Model file for the job. Use its own axes, mm. Coordinates: 2 decimals unless noted, no trailing zeros. Order: outer loops, then holes, each group sorted by start corner. A loop starts at its lowest first (then second) coordinate and runs counter-clockwise, first axis right, second up. Notation, with made-up numbers: (-19.5, -11.75) -> (8.5, -11.75) arc R35 ccw to (8.5, 25.25) -> close; hole circle Ø5 at (86, 32). An arc over 180 degrees is marked (long way). Write item = value, one per line. Start each with the question number.
Q1. Cut at D-D, the plane y = 1.45. Give the number of separate pieces and of enclosed holes in the cut face, plus the area to 3 significant figures.
Q2. Cut at A-A, the plane x = -11.5. List the corners of the cut face in (y, z).
Q3. Flat gauge pin, fed straight in: pin 1 (1.8 mm diameter, centred on x = -29.13, z = -12, fed in from -Y). Where does the tip first touch, or does it go through?
Q4. Cut at C-C, the plane z = 5.25. List the corners of the cut face in (x, y).
Q5. Wall check: line 1 (Z direction, x = 13, y = 0.85); line 2 (X direction, y = 1.7, z = 7); line 3 (X direction, y = 0.65, z = 9.25). Give the ranges that are in metal, low to high. Write a range as from..to.
Q6. Cut at B-B, the plane z = 12. List the corners of the cut face in (x, y).
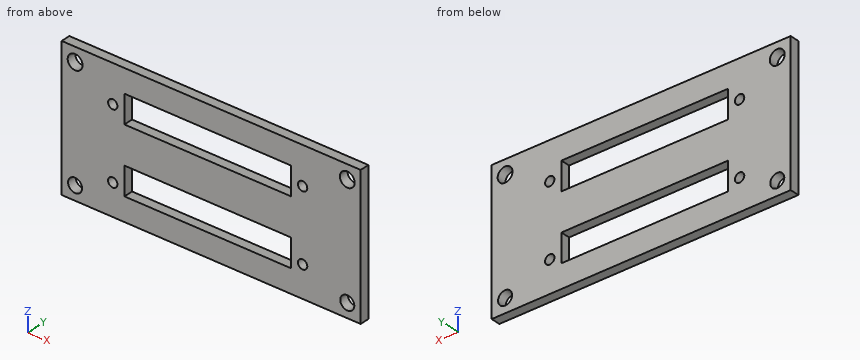
from build123d import *

# Parameters (mm, degrees)
SKETCH2_W           = 64
SKETCH2_H           = 30
SKETCH2_R           = 1.589304783
SKETCH2_R_2         = 1.5
BOSS_EXTRUDE1_DEPTH = 2
SKETCH3_R           = 1
SKETCH3_W           = 35.640445049
SKETCH3_H           = 6
CUT_EXTRUDE1_DEPTH  = 2


with BuildPart() as part:
    # Sketch2 → Boss-Extrude1 (new body)
    with BuildSketch(Plane(origin=(0, 0, 0), x_dir=(1, 0, 0), z_dir=(0, 1, 0))):
        Rectangle(SKETCH2_W, SKETCH2_H)
        with Locations(Location((-29.13, -12, 0), (0, 0, 270))):
            Circle(SKETCH2_R, mode=Mode.SUBTRACT)
        with Locations(Location((-29.134119409, 12, 0), (0, 0, 270))):
            Circle(SKETCH2_R_2, mode=Mode.SUBTRACT)
        with Locations(Location((29.13, -12, 0), (0, 0, 90))):
            Circle(SKETCH2_R, mode=Mode.SUBTRACT)
        with Locations(Location((29.134119409, 12, 0), (0, 0, 90))):
            Circle(SKETCH2_R_2, mode=Mode.SUBTRACT)
    extrude(amount=BOSS_EXTRUDE1_DEPTH)

    # Sketch3 → Cut-Extrude1 (cut)
    with BuildSketch(Plane(origin=(0, 2, 0), x_dir=(1, 0, 0), z_dir=(0, 1, 0))):
        with Locations(Location((-21.068550994, 8.267170413, 0), (0, 0, 270))):
            Circle(SKETCH3_R)
        with Locations(Location((19.571449006, 8.267170413, 0), (0, 0, 90))):
            Circle(SKETCH3_R)
        with Locations(Location((19.571449006, -6.952829587, 0), (0, 0, 270))):
            Circle(SKETCH3_R)
        with Locations(Location((-21.068550994, -6.952829587, 0), (0, 0, 90))):
            Circle(SKETCH3_R)
        with Locations((-0.74832847, -7)):
            Rectangle(SKETCH3_W, SKETCH3_H)
        with Locations((-0.74832847, 7)):
            Rectangle(SKETCH3_W, SKETCH3_H)
    extrude(amount=-CUT_EXTRUDE1_DEPTH, mode=Mode.SUBTRACT)


solid = part.part
Here are the results:
q1.separate_pieces = 1
q1.enclosed_holes = 10
q1.area = 1,450 mm²
q2.outline = (0, -15) -> (2, -15) -> (2, -10) -> (0, -10) -> close; (0, -4) -> (2, -4) -> (2, 4) -> (0, 4) -> close; (0, 10) -> (2, 10) -> (2, 15) -> (0, 15) -> close
q3.pin_1 = through
q4.outline = (-32, 0) -> (-18.57, 0) -> (-18.57, 2) -> (-32, 2) -> close; (17.07, 0) -> (32, 0) -> (32, 2) -> (17.07, 2) -> close
q5.line_1 = -15..-10, -4..4, 10..15
q5.line_2 = -32..-22.07, -20.07..-18.57, 17.07..18.57, 20.57..32
q5.line_3 = -32..-18.57, 17.07..32
q6.outline = (-32, 0) -> (-30.72, 0) -> (-30.72, 2) -> (-32, 2) -> close; (-27.54, 0) -> (27.54, 0) -> (27.54, 2) -> (-27.54, 2) -> close; (30.72, 0) -> (32, 0) -> (32, 2) -> (30.72, 2) -> close
